from build123d import *

# Parameters (mm, degrees)
F1_DEPTH = 63.5
F2_DEPTH = 25.4
F3_DEPTH = 7.9375
F5_R     = 6.35
F7_D     = 19.05


with BuildPart() as f1:
    # F0 (on Front) → F1 (new body, symmetric)
    with BuildSketch(Plane.XZ):
        Polygon((-41.275, -9.525), (41.275, -9.525), (41.275, 9.525), (22.225, 9.525), (-41.275, 9.525), align=None)
    extrude(amount=F1_DEPTH, both=True)

    # F0 (on Front) → F2 (join, symmetric)
    with BuildSketch(Plane.XZ):
        with BuildLine():
            Line((22.225, 9.525), (41.275, 9.525))
            Line((41.275, 9.525), (41.275, 27.0002))
            ThreePointArc((41.275, 27.0002), (45.92468, 38.22552), (57.15, 42.8752))
            Line((57.15, 42.8752), (60.325, 42.8752))
            Line((60.325, 42.8752), (60.325, 61.9252))
            Line((60.325, 61.9252), (57.15, 61.9252))
            ThreePointArc((57.15, 61.9252), (32.454296, 51.695904), (22.225, 27.0002))
            Line((22.225, 27.0002), (22.225, 9.525))
        make_face()
        Polygon((85.725, 61.9252), (60.325, 61.9252), (60.325, 42.8752), (85.725, 42.8752), (85.725, 52.3875), align=None)
    extrude(amount=F2_DEPTH, both=True)

    # F0 (on Front) → F3 (join, symmetric)
    with BuildSketch(Plane.XZ):
        with BuildLine():
            add(Edge.make_bspline(
                [(-41.275, 9.525), (-41.461322, 33.962093), (16.207486, 62.256526), (57.15, 61.9252)],
                knots=[0, 0, 0, 0, 111.504536, 111.504536, 111.504536, 111.504536], degree=3))
            Line((-41.275, 9.525), (22.225, 9.525))
            Line((22.225, 9.525), (22.225, 27.0002))
            ThreePointArc((22.225, 27.0002), (32.454296, 51.695904), (57.15, 61.9252))
        make_face()
    extrude(amount=F3_DEPTH, both=True)

    # F0 (on Front) → F4 (revolve)
    with BuildSketch(Plane.XZ):
        Polygon((85.725, 66.675), (85.725, 61.9252), (85.725, 52.3875), (85.725, 42.8752), (85.725, 38.1), (111.125, 38.1), (111.125, 66.675), align=None)
    revolve(axis=Axis((85.725, 0, 57.15635), (0, 0, 1)))

    # F5
    f5_edges = [f1.edges().sort_by_distance(p)[0] for p in [
        (41.275, -63.5, 0),
        (-41.275, -63.5, 0),
        (41.275, 63.5, 0),
        (-41.275, 63.5, 0),
    ]]
    fillet(f5_edges, radius=F5_R)

    # F7 (through all)
    with Locations(Plane.XY.offset(66.675)):
        with Locations((85.725, 0)):
            Hole(F7_D / 2)


solid = f1.part
Can you work these out from the model? Positions are in its coordinate system, mm. A direction names the side the tool comes from. Coordinates: 2 decimals unless noted, no trailing zeros. Order: outer loops, then holes, each group sorted by start corner. A loop starts at its lowest first (then second) coordinate and runs counter-clockwise, first axis right, second up. Notation, with made-up numbers: M -22,73.5 L -12,73.5 A30 ccw -12,105.5 Z; hole C 17.25,-23.5 d3. An arc over 180 degrees is marked long. Write item = value, one per line.
(1) I need wall thicknesses on line 1 along X through (y, z) = (1, 39); line 2 along Y through (x, z) = (16, 45); line 3 along Z through (x, y) = (102, 18) (3 decimals). Which ranges of each line are inside material? Lowest first, please. Write a range as [from, to].
Results are:
line_1 = [-17.92, 46.76], [60.34, 76.25], [95.2, 111.11]
line_2 = [-7.94, 7.94]
line_3 = [38.1, 66.675]
(2) For faces 1 (the face through (32.73, 16.55, 51.97)), 2 (the face through (46, -25.4, 42)), 3 (the face through (75, 0, 38.1)), which set-ups out of +Z, -Z, +X, -X, +Y, -Y let a thin tool reach every point of the face, with its end or its side?
Results are:
face_1 = +Z, -X, +Y
face_2 = +Z, +X, -X, -Y
face_3 = -Z, +X, +Y, -Y
(3) For pin 1 Ø4 at (x, y) = (8.5, 18.5) entering from +Z (3 decimals); pin 2 Ø14.5 at (x, y) = (73.5, -8.5) entering from -Z; pin 3 Ø14 at (y, z) = (-15, 19.5) entering from -X (3 decimals), each with a flat end and sliding along its axis, tell me the tip position at first contact or that it passes through.
Results are:
pin_1 = 9.525
pin_2 = 38.1
pin_3 = 22.225
(4) Suppose I cut it at B-B on z = 40.5. State how many separate pieces and enclosed holes the cut face has, plus the area to 3 significant figures.
Results are:
separate_pieces = 2
enclosed_holes = 1
area = 3,600 mm2
(5) If we mould it in two halves opening along Y, with no side actions, what happens to faces 4 (the face through (95.24, 0.42, 52.19)), 5 (the face through (39.464, -61.59, 0.133)), 6 (the face through (39.464, 61.59, 0.133)), 7 (the face through (45.8, -0.4, 38.1))? For each: pulls with the +Y half, pulls with the -Y half, needs draft (parallel to the pull), parting line crosses it, or undercut.
Results are:
face_4 = undercut
face_5 = pulls with the -Y half
face_6 = pulls with the +Y half
face_7 = needs draft
(6) Suppose I cut it at A-A on x = 92. Please give me the cut outline in (y, z) (3 decimals), plus the area to 3 significant figures.
Results are:
outline = M -24.613,38.1 L -7.166,38.1 L -7.166,66.675 L -24.613,66.675 Z; M 7.166,38.1 L 24.613,38.1 L 24.613,66.675 L 7.166,66.675 Z
area = 997 mm2
